Work out the finished part from the listing and answer in its coordinate system (mm). A direction names the side the tool comes from. Give positions to 0.01 mm unless a question says otherwise; leave off trailing zeros. Order: outer loops, then holes, each group sorted by start corner. A loop starts at its lowest first (then second) coordinate and runs counter-clockwise, first axis right, second up. Notation, with made-up numbers: (84, 26) - (128, 26) arc R25 ccw to (128, 47) - close; hole circle Ø3 at (70, -1.75). An arc over 180 degrees is marked (long way). Write each question's results on one line, items separated by ' | '.
from build123d import *

# Parameters (mm, degrees)
BASE_EXTRUDE_DEPTH = 12.7


with BuildPart() as part:
    # Sketch1 → Base-Extrude (new, symmetric)
    with BuildSketch(Plane.XY):
        with BuildLine():
            Line((17.6403, 16.339286512), (19.729882578, 19.063533504))
            ThreePointArc((19.729882578, 19.063533504), (19.156045845, 20.609744632), (17.6403, 21.2598))
            Line((17.6403, 21.2598), (14.70327367, 21.2598))
            ThreePointArc((14.70327367, 21.2598), (13.223883481, 20.647016519), (12.6111, 19.16762633))
            Line((12.6111, 19.16762633), (12.6111, 15.61465))
            Line((12.6111, 15.61465), (11.1125, 15.61465))
            Line((11.1125, 15.61465), (11.1125, 19.16762633))
            ThreePointArc((11.1125, 19.16762633), (12.164213258, 21.706686742), (14.70327367, 22.7584))
            Line((14.70327367, 22.7584), (17.6403, 22.7584))
            ThreePointArc((17.6403, 22.7584), (20.415434554, 21.446284653), (21.162428673, 18.4688666))
            Line((21.162428673, 18.4688666), (19.1389, 15.830735923))
            Line((19.1389, 15.830735923), (19.1389, 10.749129415))
            Line((19.1389, 10.749129415), (20.6375, 9.0662125))
            Line((20.6375, 9.0662125), (20.6375, -4.8244125))
            Line((20.6375, -4.8244125), (19.1389, -6.507329415))
            Line((19.1389, -6.507329415), (19.1389, -13.358784555))
            Line((19.1389, -13.358784555), (20.553458003, -14.773342558))
            ThreePointArc((20.553458003, -14.773342558), (18.729942105, -18.270236732), (15.019825564, -16.932883251))
            ThreePointArc((15.019825564, -16.932883251), (13.000752562, -16.523120627), (12.480559153, -18.5166))
            Line((12.480559153, -18.5166), (-12.480559153, -18.5166))
            ThreePointArc((-12.480559153, -18.5166), (-13.000752562, -16.523120627), (-15.019825564, -16.932883251))
            ThreePointArc((-15.019825564, -16.932883251), (-18.729942105, -18.270236732), (-20.553458003, -14.773342558))
            Line((-20.553458003, -14.773342558), (-19.1389, -13.358784555))
            Line((-19.1389, -13.358784555), (-19.1389, -6.507329415))
            Line((-19.1389, -6.507329415), (-20.6375, -4.8244125))
            Line((-20.6375, -4.8244125), (-20.6375, 9.0662125))
            Line((-20.6375, 9.0662125), (-19.1389, 10.749129415))
            Line((-19.1389, 10.749129415), (-19.1389, 15.830735923))
            Line((-19.1389, 15.830735923), (-21.162428673, 18.4688666))
            ThreePointArc((-21.162428673, 18.4688666), (-20.415434554, 21.446284653), (-17.6403, 22.7584))
            Line((-17.6403, 22.7584), (-14.70327367, 22.7584))
            ThreePointArc((-14.70327367, 22.7584), (-12.164213258, 21.706686742), (-11.1125, 19.16762633))
            Line((-11.1125, 19.16762633), (-11.1125, 15.61465))
            Line((-11.1125, 15.61465), (-12.6111, 15.61465))
            Line((-12.6111, 15.61465), (-12.6111, 19.16762633))
            ThreePointArc((-12.6111, 19.16762633), (-13.223883481, 20.647016519), (-14.70327367, 21.2598))
            Line((-14.70327367, 21.2598), (-17.6403, 21.2598))
            ThreePointArc((-17.6403, 21.2598), (-19.156045845, 20.609744632), (-19.729882578, 19.063533504))
            Line((-19.729882578, 19.063533504), (-17.6403, 16.339286512))
            Line((-17.6403, 16.339286512), (-17.6403, 10.17860201))
            Line((-17.6403, 10.17860201), (-19.1389, 8.495685095))
            Line((-19.1389, 8.495685095), (-19.1389, -4.253885095))
            Line((-19.1389, -4.253885095), (-17.6403, -5.93680201))
            Line((-17.6403, -5.93680201), (-17.6403, -13.979525))
            Line((-17.6403, -13.979525), (-19.1389, -15.478125))
            ThreePointArc((-19.1389, -15.478125), (-18.092238669, -16.906954381), (-16.414285827, -16.33992034))
            ThreePointArc((-16.414285827, -16.33992034), (-13.428073412, -14.819877156), (-10.898992189, -17.018))
            Line((-10.898992189, -17.018), (10.898992189, -17.018))
            ThreePointArc((10.898992189, -17.018), (13.323359075, -14.834630878), (16.30518861, -16.15877141))
            ThreePointArc((16.30518861, -16.15877141), (17.990302879, -16.935279743), (19.1389, -15.478125))
            Line((19.1389, -15.478125), (17.6403, -13.979525))
            Line((17.6403, -13.979525), (17.6403, -5.93680201))
            Line((17.6403, -5.93680201), (19.1389, -4.253885095))
            Line((19.1389, -4.253885095), (19.1389, 8.495685095))
            Line((19.1389, 8.495685095), (17.6403, 10.17860201))
            Line((17.6403, 10.17860201), (17.6403, 16.339286512))
        make_face()
    base_extrude = extrude(amount=BASE_EXTRUDE_DEPTH, both=True)

    # Mirror1: Base-Extrude across plane
    add(base_extrude.mirror(Plane(origin=(0, -18.5166, 0), x_dir=(0, 0, 1), z_dir=(0, -1, 0))))


solid = part.part
1. A cutting plane is placed at A-A, the plane y = -2.5. Write down the section's boundary in (x, z), then the cut area to 3 significant figures.
Answer list:
outline: (-20.64, -12.7) - (-19.14, -12.7) - (-19.14, 12.7) - (-20.64, 12.7) - close; (19.14, -12.7) - (20.64, -12.7) - (20.64, 12.7) - (19.14, 12.7) - close | area: 76.1 mm^2
2. Straight lines are drawn through the part: line 1 (X direction, y = 5.5, z = -1.5); line 2 (X direction, y = -20.5, z = 3.5); line 3 (X direction, y = -28, z = 5). For each, find the intervals that lie inside material, in ascending order. Write a range as [from, to].
Answer list:
line 1: [-20.64, -19.14], [19.14, 20.64] | line 2: [-20.45, -18.7], [-16.58, -14.6], [-12.98, -11.08], [11.08, 12.98], [14.6, 16.58], [18.7, 20.45] | line 3: [-19.14, -17.64], [17.64, 19.14]
3. A tool of negligible diameter and unlimited length cuts with its end or side. For faces 1 (the face through (-19.899, 9.896, 0.178)), 2 (the face through (-18.117, -20.134, 0.178)), 3 (the face through (19.139, 13, 0)), from which of +Z, -Z, +X, -X, +Y, -Y can it reach the whole face along a straight path? Write none if from no direction.
Answer list:
face 1: +Z, -Z, -X | face 2: +Z, -Z | face 3: +Z, -Z, +X
4. Determine the mould class of faces 4 (the face through (0, -20.015, 0)), 5 (the face through (18.4, -14.74, 0.18)), 6 (the face through (11.112, -54, 0)) for opening direction Y: +Y half, -Y half, draft (parallel to the pull), parting line (faces both ways), or undercut.
Answer list:
face 4: -Y half | face 5: undercut | face 6: draft
5. A cutting plane is placed at B-B, the plane x = -13.5. Write down the section's boundary in (y, z).
Answer list:
outline: (-59.58, -12.7) - (-57.91, -12.7) - (-57.91, 12.7) - (-59.58, 12.7) - close; (-22.22, -12.7) - (-20.71, -12.7) - (-20.71, 12.7) - (-22.22, 12.7) - close; (-16.33, -12.7) - (-14.81, -12.7) - (-14.81, 12.7) - (-16.33, 12.7) - close; (20.88, -12.7) - (22.55, -12.7) - (22.55, 12.7) - (20.88, 12.7) - close
6. Given P1, Ø5, axis at y = 13.5, z = 4.5, coming from the -X side; P2, Ø10, axis at y = -42, z = -1.5, coming from the -X side; P3, Ø10, axis at y = 13, z = -1, coming from the +X side, each flat-ended and moving along its own axis, determine where each tip first touches the part or whether it passes through.
Answer list:
P1: x = -19.27 | P2: x = -20.64 | P3: x = 20.8
7. A cutting plane is placed at C-C, the plane x = -4. Write down the section's boundary in (y, z), then the cut area to 3 significant figures.
Answer list:
outline: (-20.02, -12.7) - (-17.02, -12.7) - (-17.02, 12.7) - (-20.02, 12.7) - close | area: 76.1 mm^2
